from build123d import *

# Parameters (mm, degrees)
SKETCH_1_R      = 6
SKETCH_1_R_2    = 1.5
EXTRUDE_1_DEPTH = 2
CHAMFER_1_SIZE  = 0.1


with BuildPart() as part:
    # 草图1 → 凸台-拉伸1 (new, symmetric)
    with BuildSketch(Plane.XY):
        Circle(SKETCH_1_R)
        Circle(SKETCH_1_R_2, mode=Mode.SUBTRACT)
    extrude(amount=EXTRUDE_1_DEPTH, both=True)

    # 切除-扫描1: sweep along a curve in space
    with BuildLine() as sweep_1_path:
        ThreePointArc((6, 0, -2), (4.242640687, 4.242640687, -2), (0, 6, -2))
        ThreePointArc((0, 6, -2), (-4.242640687, 4.242640687, -2), (-6, 0, -2))
        ThreePointArc((-6, 0, -2), (-4.242640687, -4.242640687, -2), (0, -6, -2))
        ThreePointArc((0, -6, -2), (4.242640687, -4.242640687, -2), (6, 0, -2))
    # 草图2 → 切除-扫描1 (sweep, cut)
    with BuildSketch(Plane(origin=(0, 0, 0), x_dir=(0, 0, -1), z_dir=(1, 0, 0))):
        with BuildLine():
            Line((-1.25, 6), (1.25, 6))
            ThreePointArc((1.25, 6), (0, 5.1), (-1.25, 6))
        make_face()
    sweep(path=sweep_1_path.line, mode=Mode.SUBTRACT)

    # 倒角1
    chamfer_1_edges = [part.edges().sort_by_distance(p)[0] for p in [
        (-6, 0, -2),
        (-6, 0, 2),
        (-1.5, 0, -2),
        (-1.5, 0, 2),
    ]]
    chamfer(chamfer_1_edges, length=CHAMFER_1_SIZE)


solid = part.part
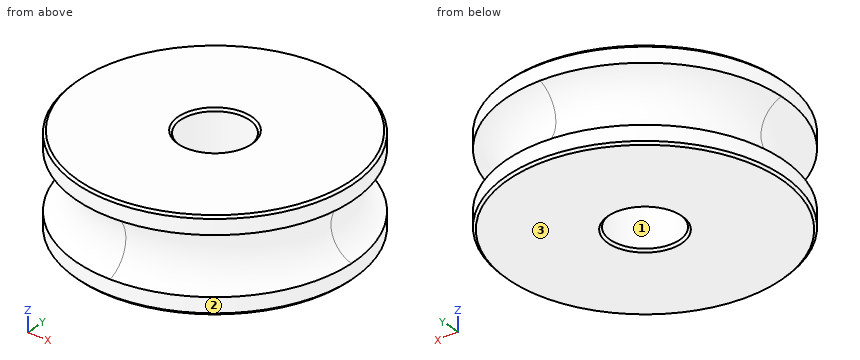
Can you work these out from the model? Positions are in its coordinate system, mm. Face numbers are marked on the shaded views. Coordinates: 2 decimals unless noted, no trailing zeros. Write each loop counter-clockwise with the first axis right and the second up, starting at its lowest first coordinate (ties: lowest second). Pieces come first, ordered by that corner, then holes. Notation, with made-up numbers: (-5, 2) -> (50, 2) arc R33 ccw to (50, 33) -> close; hole circle Ø9 at (45.25, -1.5). An arc over 180 degrees is marked (long way). Write each question's results on one line, items separated by ' | '. Start each with the question number.
Q1. Imagine slicing it at C-C (z = 1.7). Write out the boundary of the cut face in (x, y).
Q2. Imagine slicing it at B-B (z = -0.8). Write out the boundary of the cut face in (x, y), then the cut area to 3 significant figures.
Q3. If I drill on probe 1 along Y at (x, z) = (-1, -0.35); probe 2 along X at (y, z) = (0.25, 0.2); probe 3 along Y at (x, z) = (-1.25, -0.7), over which ranges is the centre line in solid material (lowest first)?
Q4. Imagine slicing it at A-A (z = 0.45). Write out the boundary of the cut face in (x, y), then the cut area to 3 significant figures.
Q5. I'm going to push flat-ended pins straight in: pin 1 (1.5 mm diameter, centred on y = 2, z = 1.5, fed in from +X); pin 2 (1 mm diameter, centred on y = 3.5, z = 1, fed in from +X). Where does each tip first touch, or does it pass through?
Q6. We'd pull the mould along X, two halves only. Please class the marked faces 1, 2 and 3: +X half, -X half, draft (parallel to the pull), parting line (faces both ways), or undercut.
Taken from the geometry:
1) outline: circle Ø12 at (0, 0); hole circle Ø3 at (0, 0)
2) outline: circle Ø10.74 at (0, 0); hole circle Ø3 at (0, 0) | area: 83.5 mm^2
3) probe 1: y = -5.05 to -1.12, 1.12 to 5.05 | probe 2: x = -5.11 to -1.48, 1.48 to 5.11 | probe 3: y = -5.15 to -0.83, 0.83 to 5.15
4) outline: circle Ø10.36 at (0, 0); hole circle Ø3 at (0, 0) | area: 77.2 mm^2
5) pin 1: stops at x = 5.87 | pin 2: stops at x = 5.16
6) face 1: undercut | face 2: parting line | face 3: draft
